```python
from build123d import *

# Parameters (mm, degrees)
SKETCH1_W           = 80
SKETCH1_H           = 7
BOSS_EXTRUDE1_DEPTH = 30
SKETCH2_R           = 3
SKETCH2_R_2         = 2
BOSS_EXTRUDE2_DEPTH = 20
SKETCH7_W           = 20
SKETCH7_H           = 20
CUT_EXTRUDE1_DEPTH  = 52.941693496
SKETCH9_R           = 4.1
CUT_EXTRUDE2_DEPTH  = 68.885232888
SKETCH11_R          = 4
SKETCH11_R_2        = 2
BOSS_EXTRUDE6_DEPTH = 20
FILLET1_R           = 5
FILLET2_R           = 4
SKETCH14_W          = 40
SKETCH14_H          = 2
BOSS_EXTRUDE8_DEPTH = 30
FILLET4_START       = 8
FILLET4_DEPTH       = 2
FILLET4_2_DEPTH     = 2
SKETCH15_R          = 2
CUT_EXTRUDE3_DEPTH  = 58.907259499
SKETCH16_W          = 20.48
SKETCH16_H          = 5
SKETCH16_W_2        = 24.48
CUT_EXTRUDE4_DEPTH  = 58.907259499
SKETCH11_2_R        = 4
SKETCH11_2_R_2      = 2
CUT_EXTRUDE5_DEPTH  = 10
CUT_EXTRUDE6_REACH  = 61.965
SKETCH17_R          = 2
CUT_EXTRUDE7_START  = -3
CUT_EXTRUDE7_DEPTH  = 3
FILLET5_R           = 3


with BuildPart() as part:
    # Sketch1 → Boss-Extrude1 (new body)
    with BuildSketch(Plane(origin=(0, 0, 0), x_dir=(1, 0, 0), z_dir=(0, 1, 0))):
        with Locations((1.820324284, 6.911764706)):
            Rectangle(SKETCH1_W, SKETCH1_H)
    extrude(amount=BOSS_EXTRUDE1_DEPTH)

    # Sketch2 → Boss-Extrude2 (add)
    # profile 1 of 2: a face of its own
    with BuildSketch(Plane.XZ):
        with Locations(Location((-33.679675716, -6.911764706, 0), (0, 0, 270))):
            Circle(SKETCH2_R)
        with Locations(Location((-33.679675716, -6.911764706, 0), (0, 0, 270))):
            Circle(SKETCH2_R_2, mode=Mode.SUBTRACT)
    # profile 2 of 2: a face of its own
    with BuildSketch(Plane.XZ):
        with Locations(Location((37.320324284, -6.911764706, 0), (0, 0, 270))):
            Circle(SKETCH2_R)
        with Locations(Location((37.320324284, -6.911764706, 0), (0, 0, 270))):
            Circle(SKETCH2_R_2, mode=Mode.SUBTRACT)
    extrude(amount=BOSS_EXTRUDE2_DEPTH)

    # Sketch7 → Cut-Extrude1 (cut, through all)
    with BuildSketch(Plane(origin=(0, 0, -10.411764706), x_dir=(-1, 0, 0), z_dir=(0, 0, -1))):
        with Locations((-31.820324284, 20)):
            Rectangle(SKETCH7_W, SKETCH7_H)
        with Locations((28.179675716, 20)):
            Rectangle(SKETCH7_W, SKETCH7_H)
    extrude(amount=-CUT_EXTRUDE1_DEPTH, mode=Mode.SUBTRACT)

    # Sketch9 → Cut-Extrude2 (cut, through all)
    with BuildSketch(Plane.ZY.offset(18.179675716)):
        with Locations((-6.911764706, 30)):
            Circle(SKETCH9_R)
    extrude(amount=-CUT_EXTRUDE2_DEPTH, mode=Mode.SUBTRACT)

    # Sketch11 → Boss-Extrude6 (add)
    with BuildSketch(Plane(origin=(21.820324284, 0, 0), x_dir=(0, 0, -1), z_dir=(1, 0, 0))):
        with Locations((6.911764706, 29.801076023)):
            Circle(SKETCH11_R)
        with Locations((6.911764706, 29.801076023)):
            Circle(SKETCH11_R_2, mode=Mode.SUBTRACT)
    extrude(amount=-BOSS_EXTRUDE6_DEPTH)

    # Fillet1
    fillet1_edges = [part.edges().sort_by_distance(p)[0] for p in [
        (21.820324284, 10, -6.911764706),
        (-18.179675716, 10, -6.911764706),
    ]]
    fillet(fillet1_edges, radius=FILLET1_R)

    # Fillet2
    # the kernel refuses this fillet: 4 mm, written as the material it takes off along each edge
    with BuildSketch(Plane(origin=(41.820324284, -10, -10.411764706), x_dir=(-1, 0, 0), z_dir=(0, 1, 0)), Plane(origin=(41.820324284, -10, -3.411764706), x_dir=(0, 0, -1), z_dir=(0, 1, 0))) as fillet2_piece_1:
        with BuildLine():
            CenterArc((FILLET2_R, FILLET2_R), FILLET2_R, 180, 90)
            Line((0, FILLET2_R), (0, 0))
            Line((0, 0), (FILLET2_R, 0))
        make_face()
    extrude(amount=30, mode=Mode.SUBTRACT)
    with BuildSketch(Plane(origin=(-38.179675716, -10, -3.411764706), x_dir=(0, 0, -1), z_dir=(0, 1, 0)), Plane(origin=(-38.179675716, -10, -10.411764706), x_dir=(1, 0, 0), z_dir=(0, 1, 0))) as fillet2_piece_2:
        with BuildLine():
            CenterArc((FILLET2_R, -FILLET2_R), FILLET2_R, 90, 90)
            Line((0, -FILLET2_R), (0, 0))
            Line((0, 0), (FILLET2_R, 0))
        make_face()
    extrude(amount=30, mode=Mode.SUBTRACT)

    # Sketch14 → Boss-Extrude8 (add)
    with BuildSketch(Plane.XY.offset(-3.411764706)):
        with Locations((1.820324284, 9)):
            Rectangle(SKETCH14_W, SKETCH14_H)
    extrude(amount=BOSS_EXTRUDE8_DEPTH)

    # Fillet4: read off the stored shape, not the designer's step
    # Fillet4 outline → Fillet4 (cut)
    with BuildSketch(Plane(origin=(0, 0, 0), x_dir=(1, 0, 0), z_dir=(0, 1, 0)).offset(FILLET4_START)):
        with BuildLine():
            Line((-18.179675716, -26.588235294), (-13.179675716, -26.588235294))
            ThreePointArc((-13.179675716, -26.588235294), (-16.715209622, -25.1237692), (-18.179675716, -21.588235294))
            Line((-18.179675716, -21.588235294), (-18.179675716, -26.588235294))
        make_face()
        with BuildLine():
            ThreePointArc((21.820324284, -21.588235294), (20.35585819, -25.123769199), (16.820324284, -26.588235294))
            Line((16.820324284, -26.588235294), (21.820324284, -26.588235294))
            Line((21.820324284, -26.588235294), (21.820324284, -21.588235294))
        make_face()
    extrude(amount=FILLET4_DEPTH, mode=Mode.SUBTRACT)

    # Fillet4 2 outline → Fillet4 2 (add)
    with BuildSketch(Plane(origin=(0, 0, 0), x_dir=(1, 0, 0), z_dir=(0, 1, 0)).offset(FILLET4_START)):
        with BuildLine():
            ThreePointArc((-23.179675716, 3.411764706), (-19.64414181, 1.947298611), (-18.179675716, -1.588235294))
            Line((-18.179675716, -1.588235294), (-18.179675716, 3.411764706))
            Line((-18.179675716, 3.411764706), (-23.179675716, 3.411764706))
        make_face()
        with BuildLine():
            Line((21.820324284, 3.411764706), (21.820324284, -1.588235294))
            ThreePointArc((21.820324284, -1.588235294), (23.284790378, 1.947298612), (26.820324284, 3.411764706))
            Line((26.820324284, 3.411764706), (21.820324284, 3.411764706))
        make_face()
    extrude(amount=FILLET4_2_DEPTH)

    # Sketch15 → Cut-Extrude3 (cut, through all)
    with BuildSketch(Plane(origin=(0, 10, 0), x_dir=(1, 0, 0), z_dir=(0, 1, 0))):
        with Locations(Location((-10.889675716, -3.728235294, 0), (0, 0, 180))):
            Circle(SKETCH15_R)
        with Locations(Location((14.510324284, -3.728235294, 0), (0, 0, 180))):
            Circle(SKETCH15_R)
    extrude(amount=-CUT_EXTRUDE3_DEPTH, mode=Mode.SUBTRACT)

    # Sketch16 → Cut-Extrude4 (cut, through all)
    with BuildSketch(Plane(origin=(0, 10, 0), x_dir=(1, 0, 0), z_dir=(0, 1, 0))):
        with Locations((1.810324284, -1.228235294)):
            Rectangle(SKETCH16_W, SKETCH16_H)
        with Locations((1.810324284, -24.088235294)):
            Rectangle(SKETCH16_W_2, SKETCH16_H)
    extrude(amount=-CUT_EXTRUDE4_DEPTH, mode=Mode.SUBTRACT)

    # Sketch11<2> → Cut-Extrude5 (cut)
    with BuildSketch(Plane(origin=(21.820324284, 0, 0), x_dir=(0, 0, -1), z_dir=(1, 0, 0))):
        with Locations((6.911764706, 29.801076023)):
            Circle(SKETCH11_2_R)
        with Locations((6.911764706, 29.801076023)):
            Circle(SKETCH11_2_R_2, mode=Mode.SUBTRACT)
    extrude(amount=-CUT_EXTRUDE5_DEPTH, mode=Mode.SUBTRACT)

    # Sketch17 → Cut-Extrude6 (cut, up to next)
    with BuildSketch(Plane.XZ, mode=Mode.PRIVATE) as cut_extrude6_sk1:
        with Locations(Location((37.320324284, -6.911764706, 0), (0, 0, 270))):
            Circle(SKETCH17_R)
    cut_extrude6_tool1 = extrude(cut_extrude6_sk1.sketch, amount=-CUT_EXTRUDE6_REACH, mode=Mode.PRIVATE) & part.part
    # Sketch17 → Cut-Extrude6 (cut, up to next)
    with BuildSketch(Plane.XZ, mode=Mode.PRIVATE) as cut_extrude6_sk2:
        with Locations((-33.679675716, -6.911764706)):
            Circle(SKETCH17_R)
    cut_extrude6_tool2 = extrude(cut_extrude6_sk2.sketch, amount=-CUT_EXTRUDE6_REACH, mode=Mode.PRIVATE) & part.part
    add(cut_extrude6_tool1.solids().sort_by_distance((37.320324, 0, -6.911765))[0], mode=Mode.SUBTRACT)
    add(cut_extrude6_tool2.solids().sort_by_distance((-33.679676, 0, -6.911765))[0], mode=Mode.SUBTRACT)

    # Sketch18 → Cut-Extrude7 (cut)
    with BuildSketch(Plane(origin=(0, 10, 0), x_dir=(1, 0, 0), z_dir=(0, 1, 0)).offset(CUT_EXTRUDE7_START)):
        with BuildLine():
            Line((37.820324284, 10.411764706), (33.320324284, 10.411764706))
            Line((33.320324284, 10.411764706), (33.320324284, 3.411764706))
            Line((33.320324284, 3.411764706), (37.820324284, 3.411764706))
            ThreePointArc((37.820324284, 3.411764706), (40.466075595, 4.411764706), (41.78895125, 6.911764706))
            ThreePointArc((41.78895125, 6.911764706), (40.466075595, 9.411764706), (37.820324284, 10.411764706))
        make_face()
        with BuildLine():
            Line((-34.179675716, 3.411764706), (-29.679675716, 3.411764706))
            Line((-29.679675716, 3.411764706), (-29.679675716, 10.411764706))
            Line((-29.679675716, 10.411764706), (-34.179675716, 10.411764706))
            ThreePointArc((-34.179675716, 10.411764706), (-36.825427028, 9.411764706), (-38.148302683, 6.911764706))
            ThreePointArc((-38.148302683, 6.911764706), (-36.825427028, 4.411764706), (-34.179675716, 3.411764706))
        make_face()
    extrude(amount=CUT_EXTRUDE7_DEPTH, mode=Mode.SUBTRACT)

    # Fillet5
    fillet5_edges = [part.edges().sort_by_distance(p)[0] for p in [
        (-29.679675716, 10, -6.911764706),
        (33.320324284, 10, -6.911764706),
    ]]
    fillet(fillet5_edges, radius=FILLET5_R - 0.0001)  # a hair under: the kernel refuses the full size


solid = part.part
```
Geometry check sheet. Reference: the model listing, model coordinates, mm. A direction names the side the tool comes from. Round coordinates to 2 decimals unless told otherwise and drop trailing zeros. Order: outer loops, then holes, each group sorted by start corner. A loop starts at its lowest first (then second) coordinate and runs counter-clockwise, first axis right, second up. Notation, with made-up numbers: (43, 82) - (93, 82) arc R22 cw to (93, 107) - close; hole circle Ø4 at (78.25, 70.25). An arc over 180 degrees is marked (long way). Use a Markdown table: item, result. Add a question column.
1) Section check A-A (x = 4). Record the cut outline in (y, z), then the cut area to 3 significant figures.
2) Gauge pin test, flat ends, axial feed: P1, Ø3, axis at x = 29.5, z = -8.5, coming from the +Y side; P2, Ø2, axis at y = 22, z = -7.5, coming from the +X side; P3, Ø3.5, axis at x = 6.5, z = -7, coming from the -Y side. Record the tip position at first contact, or that the pin passes through.
3) Section check B-B (z = 0.5). Record the cut outline in (x, y).
4) Section check C-C (x = -12). Record the cut outline in (y, z).
5) Set-up check for faces 1 (the cylindrical face through (39.85, -9.86, -8.525)), 2 (the flat face through (-10.43, 9, 24)), 3 (the flat face through (-8.43, 9, 1)): record each of +Z, -Z, +X, -X, +Y, -Y from which the full face is reachable in a straight line by a thin tool's end or side.
6) Thickness scan on line 1 along X through (y, z) = (-2, -7); line 2 along Y through (x, z) = (6, -7); line 3 along Z through (x, y) = (7, 7.5). Record the ranges inside material, lowest first.
7) Section check D-D (y = -10.5). Record the cut outline in (x, z).
8) Mould release check, pull along Y, two halves, no side actions. Record for faces 4 (the flat face through (1, 19, -3.412)), 5 (the flat face through (35, -20, -8)), 6 (the cylindrical face through (-19.68, 11.43, -6.86)): released by +Y, released by -Y, zero draft, split by the parting line, or undercut.
Established:
| question | item | result |
|---|---|---|
| 1 | outline | (0, -10.41) - (27.86, -10.41) arc R4 ccw (long way) to (27.86, -3.41) - (10, -3.41) - (10, -1.27) - (8, -1.27) - (8, -3.41) - (0, -3.41) - close; (8, 3.73) - (10, 3.73) - (10, 21.59) - (8, 21.59) - close; hole circle Ø4 at (29.8, -6.91) |
| 1 | area | 262 mm2 |
| 2 | P1 | y = 10 |
| 2 | P2 | x = 21.82 |
| 2 | P3 | y = 0 |
| 3 | outline | (-18.3, 8) - (-8.43, 8) - (-8.43, 10) - (-18.3, 10) - close; (12.05, 8) - (21.94, 8) - (21.94, 10) - (12.05, 10) - close |
| 4 | outline | (0, -10.41) - (27.86, -10.41) arc R4.1 cw to (27.86, -3.41) - (10, -3.41) - (10, 2.06) - (8, 2.06) - (8, -3.41) - (0, -3.41) - close; (8, 5.39) - (10, 5.39) - (10, 26.59) - (8, 26.59) - close |
| 5 | face 1 | -Y |
| 5 | face 2 | +Z, +Y, -Y |
| 5 | face 3 | +Y, -Y |
| 6 | line 1 | -36.68 to -35.68, -31.68 to -30.68, 34.32 to 35.32, 39.32 to 40.32 |
| 6 | line 2 | 0 to 27.8, 31.8 to 33.8 |
| 6 | line 3 | -10.41 to -3.41 |
| 7 | outline | circle Ø6 at (-33.68, -6.91); circle Ø6 at (37.32, -6.91); hole circle Ø4 at (-33.68, -6.91); hole circle Ø4 at (37.32, -6.91) |
| 8 | face 4 | undercut |
| 8 | face 5 | released by -Y |
| 8 | face 6 | released by +Y |
